Check sheet for the modelled part. Datum: model origin and axes. Units: mm. A direction names the side the tool comes from. Give positions to 0.01 mm unless a question says otherwise; leave off trailing zeros. Loops run counter-clockwise (first coordinate to the right, second up) from the corner with the lowest first, then second, coordinate; pieces in that order, holes last.
```python
from build123d import *

# Parameters (mm, degrees)
BOSS_EXTRUDE1_DEPTH = 2
BOSS_EXTRUDE2_DEPTH = 30
SKETCH3_W           = 15
SKETCH3_H           = 50
BOSS_EXTRUDE3_DEPTH = 4
BOSS_EXTRUDE4_DEPTH = 6
BOSS_EXTRUDE5_DEPTH = 14
CUT_EXTRUDE1_DEPTH  = 26
BOSS_EXTRUDE6_DEPTH = 4


with BuildPart() as part:
    # Sketch1 → Boss-Extrude1 (new body)
    with BuildSketch(Plane.XY):
        Polygon((-15, 0), (-15, 36), (15, 36), (15, 50), (15, 111), (-15, 111), (-15, 50), (-30, 50), (-30, 0), align=None)
    extrude(amount=BOSS_EXTRUDE1_DEPTH)

    # Sketch2 → Boss-Extrude2 (add)
    with BuildSketch(Plane(origin=(15, 0, 0), x_dir=(0, 0, -1), z_dir=(1, 0, 0))):
        Polygon((0, 50), (7, 71.54378476), (7, 111), (0, 111), align=None)
    extrude(amount=-BOSS_EXTRUDE2_DEPTH)

    # Sketch3 → Boss-Extrude3 (add)
    with BuildSketch(Plane(origin=(0, 0, 0), x_dir=(-1, 0, 0), z_dir=(0, 0, -1))):
        with Locations((22.5, 25)):
            Rectangle(SKETCH3_W, SKETCH3_H)
    extrude(amount=BOSS_EXTRUDE3_DEPTH)

    # Sketch4 → Boss-Extrude4 (add)
    with BuildSketch(Plane(origin=(0, 0, -4), x_dir=(-1, 0, 0), z_dir=(0, 0, -1))):
        Polygon((15, 111), (15, 50), (30, 50), (30, 0), (36, 0), (36, 47), (19, 64), (19, 111), align=None)
    extrude(amount=-BOSS_EXTRUDE4_DEPTH)

    # Sketch5 → Boss-Extrude5 (add)
    with BuildSketch(Plane(origin=(0, 0, -4), x_dir=(-1, 0, 0), z_dir=(0, 0, -1))):
        Polygon((32, 0), (32, 45.343145751), (15, 62.343145751), (15, 111), (19, 111), (19, 64), (36, 47), (36, 0), align=None)
    extrude(amount=BOSS_EXTRUDE5_DEPTH)

    # Sketch6 → Cut-Extrude1 (cut)
    with BuildSketch(Plane(origin=(0, 111, 0), x_dir=(1, 0, 0), z_dir=(0, 1, 0))):
        Polygon((15, 7), (-15, 7), (-15, 18), (-19, 18), (-19, -2), (15, -2), align=None)
    extrude(amount=-CUT_EXTRUDE1_DEPTH, mode=Mode.SUBTRACT)

    # Sketch7 → Boss-Extrude6 (add)
    with BuildSketch(Plane(origin=(15, 0, 0), x_dir=(0, 0, -1), z_dir=(1, 0, 0))):
        Polygon((7, 85), (-2, 85), (-2, 36), (0, 36), (0, 50), (7, 71.54378476), align=None)
    extrude(amount=BOSS_EXTRUDE6_DEPTH)


solid = part.part
```
(1) Access from +Z, -Z, +X, -X, +Y, -Y to the whole of each face (thin tool, end or side, straight path). Record for faces 1 (the face through (1.76, 60.62, -3.45)), 2 (the face through (-19, 75, -8)), 3 (the face through (2, 36, 1)).
(2) Section check D-D on z = -1.75. Record the boundary of the cut face in (x, y), plus the area to 3 significant figures.
(3) Section check A-A on z = -15.5. Record the boundary of the cut face in (x, y).
(4) Section check B-B on x = 8.5. Record the boundary of the cut face in (y, z).
(5) Section check C-C on y = 30. Record the boundary of the cut face in (x, z).
(6) Gauge pin test, flat ends, axial feed: pin 1 Ø0.6 at (x, z) = (-1.5, 1) entering from -Y; pin 2 Ø15.5 at (x, y) = (7.5, 45) entering from -Z; pin 3 Ø4 at (y, z) = (77.5, -8.5) entering from +X; pin 4 Ø4 at (x, y) = (-9, 65.5) entering from -Z. Record the tip position at first contact, or that the pin passes through.
(7) Material ranges on line 1 (Z direction, x = 14.5, y = 78); line 2 (X direction, y = 67.5, z = -12.25); line 3 (X direction, y = 19, z = -10.5), recorded low to high.
Computed values:
1. face 1: -Z, +X, -Y
1. face 2: +Z, -Z, -X, +Y
1. face 3: +Z, -Z, +X, -Y
2. outline: (-36, 0) - (-15, 0) - (-15, 55.39) - (19, 55.39) - (19, 85) - (-19, 85) - (-19, 64) - (-36, 47) - close
2. area: 2,290 mm2
3. outline: (-36, 0) - (-32, 0) - (-32, 45.34) - (-15, 62.34) - (-15, 85) - (-19, 85) - (-19, 64) - (-36, 47) - close
4. outline: (36, 0) - (50, 0) - (71.54, -7) - (85, -7) - (85, 2) - (36, 2) - close
5. outline: (-36, -18) - (-32, -18) - (-32, -4) - (-15, -4) - (-15, 2) - (-36, 2) - close
6. pin 1: stops at y = 36
6. pin 2: stops at z = -0.89
6. pin 3: stops at x = 19
6. pin 4: stops at z = -5.69
7. line 1: z = -7 to 2
7. line 2: x = -19 to -15
7. line 3: x = -36 to -32
